Verification items for the finished model (mm, model axes). A direction names the side the tool comes from. Coordinates: 2 decimals unless noted, no trailing zeros. Loops run counter-clockwise (first coordinate to the right, second up) from the corner with the lowest first, then second, coordinate; pieces in that order, holes last. Notation, with made-up numbers: M 76,64.5 L 92,64.5 A27 cw 92,84.5 Z; hole C 84,-27 d2. An arc over 180 degrees is marked long. Write item = value, one per line. Start each with the question number.
```python
from build123d import *

# Parameters (mm, degrees)
SKETCH_1_W          = 7.5
SKETCH_1_H          = 10
SKETCH_1_W_2        = 10
SKETCH_1_H_2        = 7
EXTRUDE_1_DEPTH     = 10
CUT_EXTRUDE_1_REACH = 25.351
SKETCH_2_R          = 1.8
CUT_EXTRUDE_2_REACH = 23.937
SKETCH_3_R          = 5.25
FILLET_1_R          = 3
CUT_EXTRUDE_4_REACH = 23.937
SKETCH_5_R          = 1.75
SKETCH_6_W          = 15
SKETCH_6_H          = 10
EXTRUDE_2_DEPTH     = 93.8
SKETCH_7_W          = 21
SKETCH_7_H          = 78.8
EXTRUDE_3_DEPTH     = 10
FILLET_2_R          = 3
SKETCH_8_W          = 15
SKETCH_8_H          = 15
CUT_EXTRUDE_5_DEPTH = 5
FILLET_3_R          = 3


with BuildPart() as part:
    # 草图1 → 凸台-拉伸1 (new body)
    with BuildSketch(Plane.XY):
        with Locations((-8.75, 0)):
            Rectangle(SKETCH_1_W, SKETCH_1_H)
        Rectangle(SKETCH_1_W_2, SKETCH_1_H)
        with Locations((0, 8.5)):
            Rectangle(SKETCH_1_W_2, SKETCH_1_H_2)
        with Locations((8.75, 0)):
            Rectangle(SKETCH_1_W, SKETCH_1_H)
        with Locations((0, -10)):
            Rectangle(SKETCH_1_W_2, SKETCH_1_H)
    extrude(amount=EXTRUDE_1_DEPTH)

    # 草图2 → 切除-拉伸1 (cut, up to next)
    with BuildSketch(Plane.XZ.offset(5), mode=Mode.PRIVATE) as cut_extrude_1_sk1:
        with Locations(Location((-9.5, 5, 0), (0, 0, 270))):
            Circle(SKETCH_2_R)
    cut_extrude_1_tool1 = extrude(cut_extrude_1_sk1.sketch, amount=-CUT_EXTRUDE_1_REACH, mode=Mode.PRIVATE) & part.part
    # 草图2 → 切除-拉伸1 (cut, up to next)
    with BuildSketch(Plane.XZ.offset(5), mode=Mode.PRIVATE) as cut_extrude_1_sk2:
        with Locations(Location((9.5, 5, 0), (0, 0, 90))):
            Circle(SKETCH_2_R)
    cut_extrude_1_tool2 = extrude(cut_extrude_1_sk2.sketch, amount=-CUT_EXTRUDE_1_REACH, mode=Mode.PRIVATE) & part.part
    add(cut_extrude_1_tool1.solids().sort_by_distance((-9.5, -5, 5))[0], mode=Mode.SUBTRACT)
    add(cut_extrude_1_tool2.solids().sort_by_distance((9.5, -5, 5))[0], mode=Mode.SUBTRACT)

    # 草图3 → 切除-拉伸2 (cut, up to next)
    with BuildSketch(Plane(origin=(0, 0, 0), x_dir=(-1, 0, 0), z_dir=(0, 0, -1)), mode=Mode.PRIVATE) as cut_extrude_2_sk1:
        Circle(SKETCH_3_R)
    cut_extrude_2_tool1 = extrude(cut_extrude_2_sk1.sketch, amount=-CUT_EXTRUDE_2_REACH, mode=Mode.PRIVATE) & part.part
    add(cut_extrude_2_tool1.solids().sort_by_distance((0, 0, 0))[0], mode=Mode.SUBTRACT)

    # 圆角1
    fillet_1_edges = [part.edges().sort_by_distance(p)[0] for p in [
        (12.5, 0, 0),
        (-12.5, 0, 0),
        (12.5, 0, 10),
        (-12.5, 0, 10),
    ]]
    fillet(fillet_1_edges, radius=FILLET_1_R)

    # 草图5 → 切除-拉伸4 (cut, up to next)
    with BuildSketch(Plane.XY.offset(10), mode=Mode.PRIVATE) as cut_extrude_4_sk1:
        with Locations((0, 8)):
            Circle(SKETCH_5_R)
    cut_extrude_4_tool1 = extrude(cut_extrude_4_sk1.sketch, amount=-CUT_EXTRUDE_4_REACH, mode=Mode.PRIVATE) & part.part
    # 草图5 → 切除-拉伸4 (cut, up to next)
    with BuildSketch(Plane.XY.offset(10), mode=Mode.PRIVATE) as cut_extrude_4_sk2:
        with Locations((0, -8)):
            Circle(SKETCH_5_R)
    cut_extrude_4_tool2 = extrude(cut_extrude_4_sk2.sketch, amount=-CUT_EXTRUDE_4_REACH, mode=Mode.PRIVATE) & part.part
    add(cut_extrude_4_tool1.solids().sort_by_distance((0, 8, 10))[0], mode=Mode.SUBTRACT)
    add(cut_extrude_4_tool2.solids().sort_by_distance((0, -8, 10))[0], mode=Mode.SUBTRACT)

    # 草图6 → 凸台-拉伸2 (add)
    with BuildSketch(Plane.XZ.offset(15)):
        with Locations((0, 5)):
            Rectangle(SKETCH_6_W, SKETCH_6_H)
    extrude(amount=EXTRUDE_2_DEPTH)

    # 草图7 → 凸台-拉伸3 (add)
    with BuildSketch(Plane(origin=(0, 0, 0), x_dir=(-1, 0, 0), z_dir=(0, 0, -1))):
        with Locations((0, -54.4)):
            Rectangle(SKETCH_7_W, SKETCH_7_H)
    extrude(amount=-EXTRUDE_3_DEPTH)

    # 圆角2
    fillet_2_edges = [part.edges().sort_by_distance(p)[0] for p in [
        (-10.5, -54.4, 0),
        (10.5, -54.4, 0),
    ]]
    fillet(fillet_2_edges, radius=FILLET_2_R)

    # 草图8 → 切除-拉伸5 (cut)
    with BuildSketch(Plane(origin=(0, 0, 0), x_dir=(-1, 0, 0), z_dir=(0, 0, -1))):
        with Locations((0, -101.3)):
            Rectangle(SKETCH_8_W, SKETCH_8_H)
    extrude(amount=-CUT_EXTRUDE_5_DEPTH, mode=Mode.SUBTRACT)

    # 圆角3
    fillet_3_edges = [part.edges().sort_by_distance(p)[0] for p in [
        (-5, 12, 5),
        (5, 12, 5),
    ]]
    fillet(fillet_3_edges, radius=FILLET_3_R)


solid = part.part
```
Q1. Set-up check for faces 4 (the face through (-7.5, -101, 7)), 5 (the face through (-7, -5, 5)), 6 (the face through (-5, 7, 5)), 7 (the face through (8, -15, 5)): record each of +Z, -Z, +X, -X, +Y, -Y from which the full face is reachable in a straight line by a thin tool's end or side.
Q2. Sectioned sample at D-D on z = 1.5. Record the cut outline in (x, y), plus the area to 3 significant figures.
Q3. Scan lines: L1, parallel to Y at x = 0, z = 3.5; L2, parallel to X at y = -0.25, z = 5; L3, parallel to Y at x = 0, z = 6. Record each from-to range of solid material in increasing order. Write a range as [from, to].
Q4. Sectioned sample at A-A on y = 8. Record the cut outline in (x, z), plus the area to 3 significant figures.
Q5. Mould release check, pull along X, two halves, no side actions. Record for faces 1 (the face through (11.6, 0.07, 9.14)), 2 (the face through (1.617, -8.67, 5.07)), 3 (the face through (0, -108.8, 8)): +X half, -X half, draft (parallel to the pull), parting line (faces both ways), or undercut.
Q6. Sectioned sample at B-B on x = 0. Record the cut outline in (y, z), plus the area to 3 significant figures.
Q7. Sectioned sample at C-C on x = 6.25. Record the cut outline in (y, z).
Q8. Gauge pin test, flat ends, axial feed: pin 1 (1.2 mm diameter, centred on y = 6.5, z = 3.5, fed in from +X); pin 2 (3 mm diameter, centred on y = -12.5, z = 6, fed in from -X); pin 3 (3 mm diameter, centred on x = -9.5, z = 5, fed in from +Y). Record the tip position at first contact, or that the pin passes through.
Solutions:
q1.face_4 = +Z, -Z, -X, -Y
q1.face_5 = +Z, -Z, -X
q1.face_6 = +Z, -Z, -X, +Y
q1.face_7 = +Z, -Z, +X
q2.outline = M -12.1,-5 L -5,-5 L -5,-15 L -10.1,-15 L -10.1,-93.8 L 10.1,-93.8 L 10.1,-15 L 5,-15 L 5,-5 L 12.1,-5 L 12.1,5 L 5,5 L 5,9 A3 ccw 2,12 L -2,12 A3 ccw -5,9 L -5,5 L -12.1,5 Z; hole C 0,0 d10.5; hole C 0,-8 d3.5; hole C 0,8 d3.5
q2.area = 1,890 mm²
q3.L1 = [-93.8, -9.75], [-6.25, -5.25], [5.25, 6.25], [9.75, 12]
q3.L2 = [-12.5, -11.3], [-7.7, -5.24], [5.24, 7.7], [11.3, 12.5]
q3.L3 = [-108.8, -9.75], [-6.25, -5.25], [5.25, 6.25], [9.75, 12]
q4.outline = M -5,0 L -1.75,0 L -1.75,10 L -5,10 Z; M 1.75,0 L 5,0 L 5,10 L 1.75,10 Z
q4.area = 65.0 mm²
q5.face_1 = +X half
q5.face_2 = undercut
q5.face_3 = draft
q6.outline = M -108.8,5 L -93.8,5 L -93.8,0 L -9.75,0 L -9.75,10 L -108.8,10 Z; M -6.25,0 L -5.25,0 L -5.25,10 L -6.25,10 Z; M 5.25,0 L 6.25,0 L 6.25,10 L 5.25,10 Z; M 9.75,0 L 12,0 L 12,10 L 9.75,10 Z
q6.area = 958 mm²
q7.outline = M -108.8,5 L -93.8,5 L -93.8,0 L -15,0 L -15,10 L -108.8,10 Z; M -5,0 L 5,0 L 5,10 L -5,10 Z
q8.pin_1 = 5
q8.pin_2 = -5
q8.pin_3 = -15
